Answer from the drawing. Dimensions are ordinates in mm from the lowest x, y and z of the part. Round coordinates to 2 decimals unless told otherwise and drop trailing zeros. Loops run counter-clockwise (first coordinate to the right, second up) from the corner with the lowest first, then second, coordinate; pieces in that order, holes last. Notation, with made-up numbers: (-28, 41) -> (6, 41) arc R32 cw to (6, 70) -> close; hole circle Ø1 at (42.25, 85). An arc over 180 degrees is marked (long way). One line per question, with ' | ' between items.
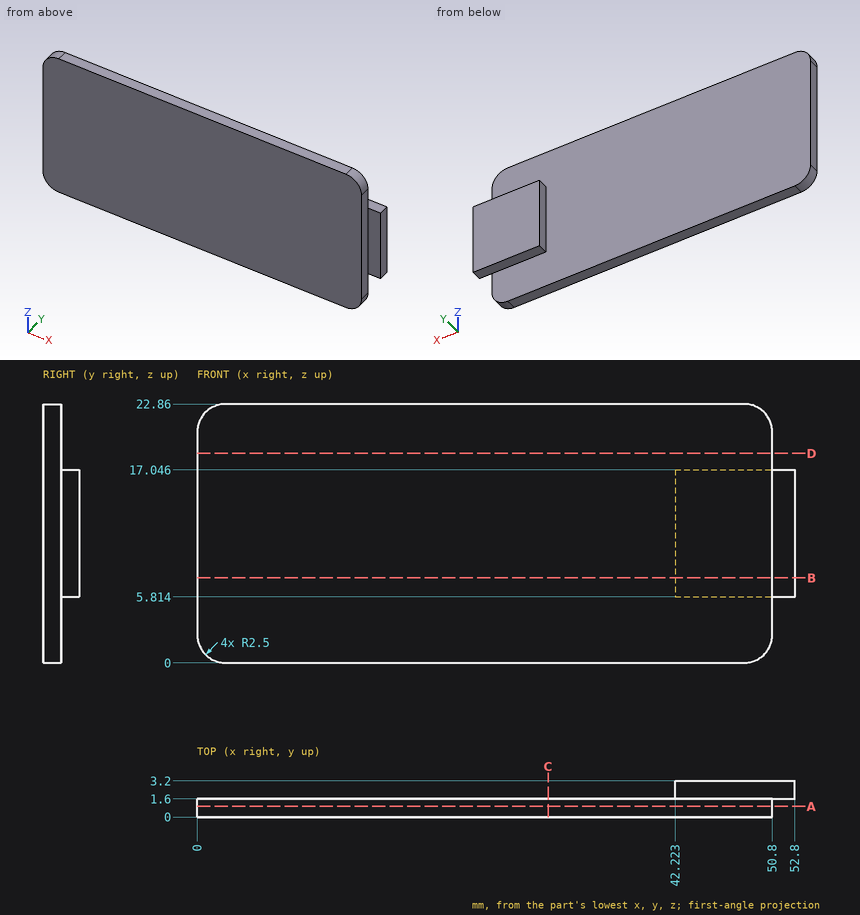
Q1. Given pin 1 Ø0.5 at (y, z) = (2.5, 9) entering from -X; pin 2 Ø0.8 at (y, z) = (1, 11.5) entering from +X; pin 3 Ø1 at (x, z) = (51.5, 10.5) entering from -Y, each flat-ended and moving along its own axis, determine where each tip first touches the part or whether it passes through.
Numbers:
pin 1: x = 42.22 | pin 2: x = 50.8 | pin 3: y = 1.6
Q2. A cutting plane is placed at A-A on y = 0.95. Give the vertices of the cut face in (x, z).
Numbers:
outline: (0, 2.5) arc R2.5 ccw to (2.5, 0) -> (48.3, 0) arc R2.5 ccw to (50.8, 2.5) -> (50.8, 20.36) arc R2.5 ccw to (48.3, 22.86) -> (2.5, 22.86) arc R2.5 ccw to (0, 20.36) -> close
Q3. Find the intervals of material crossed by line 1 (Y direction, x = 17, z = 6.75); line 2 (X direction, y = 1.7, z = 7); line 3 (X direction, y = 1.3, z = 17.25), in increasing order. Write a range as from..to.
Numbers:
line 1: 0..1.6 | line 2: 42.22..52.8 | line 3: 0..50.8
Q4. A cutting plane is placed at D-D on z = 18.5. Give the vertices of the cut face in (x, y).
Numbers:
outline: (0, 0) -> (50.8, 0) -> (50.8, 1.6) -> (0, 1.6) -> close
Q5. A cutting plane is placed at B-B on z = 7.5. Give the vertices of the cut face in (x, y).
Numbers:
outline: (0, 0) -> (50.8, 0) -> (50.8, 1.6) -> (52.8, 1.6) -> (52.8, 3.2) -> (42.22, 3.2) -> (42.22, 1.6) -> (0, 1.6) -> close
Q6. A cutting plane is placed at C-C on x = 31. Give the vertices of the cut face in (y, z).
Numbers:
outline: (0, 0) -> (1.6, 0) -> (1.6, 22.86) -> (0, 22.86) -> close
